Study the drawing (mm; zero at the part's minimum x, y, z) and answer. A direction names the side the tool comes from. Give positions to 0.01 mm unless a question says otherwise; leave off trailing zeros. Write each loop counter-clockwise with the first axis right and the second up, starting at its lowest first coordinate (ties: lowest second). Pieces come first, ordered by that corner, then holes. Notation, with made-up numbers: (-24, 28) - (13, 28) arc R27 ccw to (13, 58) - close; hole circle Ø1 at (-13.75, 57.25). An arc over 180 degrees is marked (long way). Write each question's results on one line, items separated by ' | '. Start each with the question number.
Q1. Find the intervals of material crossed by probe 1 along Y at (x, z) = (4.45, 1.9); probe 2 along Y at (x, z) = (2, 15); probe 3 along X at (y, z) = (25.65, 15.27), in increasing order.
Q2. Section A-A (z = 15.27) is taken. Determine the outline of the cut face in (x, y).
Q3. Section D-D (z = 4) is taken. Determine the outline of the cut face in (x, y).
Q4. For a pull along Y with two mould halves and no side action, classify the marked faces 1, 2 and 3 as pulls with the +Y half, pulls with the -Y half, needs draft (parallel to the pull), parting line crosses it, or undercut.
Q5. Flat-ended cylindrical pins translate along their axes: pin 1 Ø3 at (x, z) = (14, 15.27) entering from +Y; pin 2 Ø4 at (x, z) = (10.5, 14) entering from -Y; pin 3 Ø4 at (x, z) = (10, 5) entering from +Y. Find the tip coordinate at first contact, or state that the pin passes through.
Q6. For the marked faces 4, 5 and 6, determine the directions among +Z, -Z, +X, -X, +Y, -Y from which every point of the face is accessible in a straight line to the end or side of a thin tool.
Q7. Section B-B (y = 36.55) is taken. Determine the outline of the cut face in (x, z).
Q8. Section C-C (x = 4.45) is taken. Determine the outline of the cut face in (y, z).
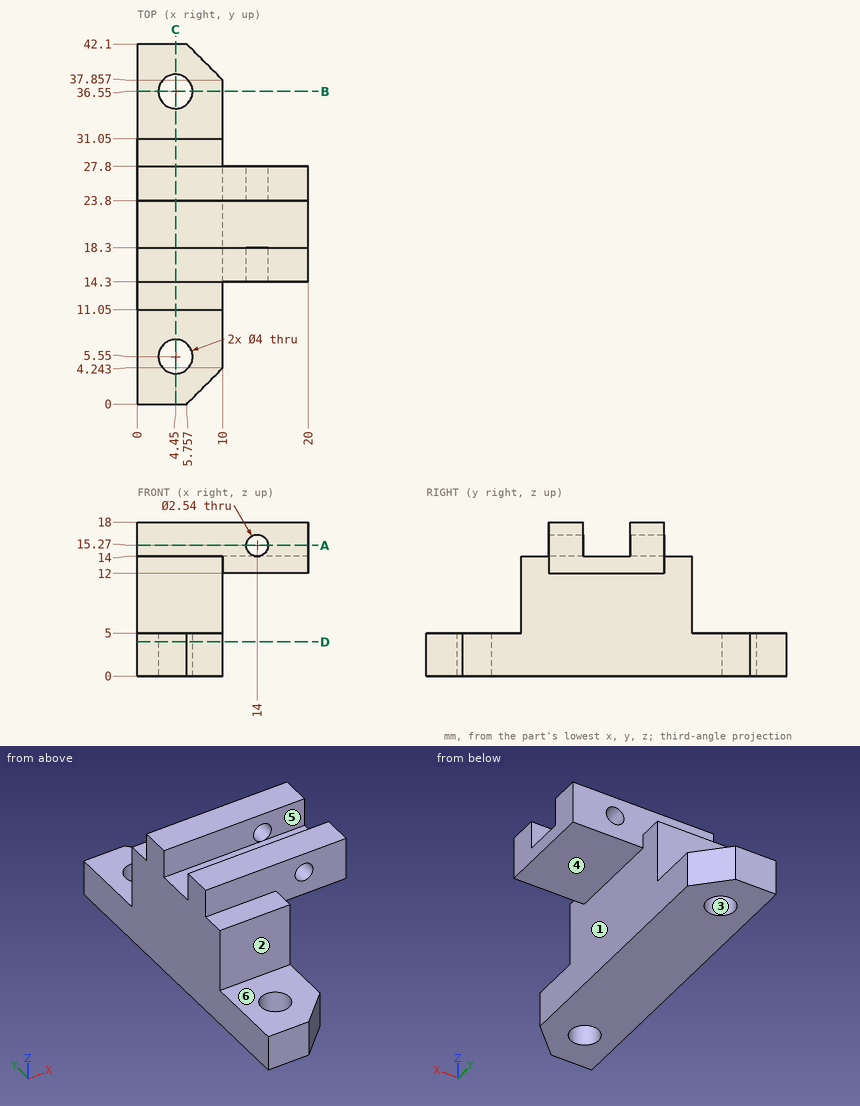
Answers below:
1) probe 1: y = 0 to 3.55, 7.55 to 34.55, 38.55 to 42.1 | probe 2: y = 14.3 to 18.3, 23.8 to 27.8 | probe 3: x = 0 to 12.73, 15.27 to 20
2) outline: (0, 14.3) - (12.73, 14.3) - (12.73, 18.3) - (0, 18.3) - close; (0, 23.8) - (12.73, 23.8) - (12.73, 27.8) - (0, 27.8) - close; (15.27, 14.3) - (20, 14.3) - (20, 18.3) - (15.27, 18.3) - close; (15.27, 23.8) - (20, 23.8) - (20, 27.8) - (15.27, 27.8) - close
3) outline: (0, 0) - (5.76, 0) - (10, 4.24) - (10, 37.86) - (5.76, 42.1) - (0, 42.1) - close; hole circle Ø4 at (4.45, 5.55); hole circle Ø4 at (4.45, 36.55)
4) face 1: needs draft | face 2: pulls with the -Y half | face 3: undercut
5) pin 1: stops at y = 27.8 | pin 2: stops at y = 11.05 | pin 3: stops at y = 39.86
6) face 4: -Z, +X, +Y, -Y | face 5: +Z, +X, -X | face 6: +Z, +X, -X, -Y
7) outline: (0, 0) - (2.45, 0) - (2.45, 5) - (0, 5) - close; (6.45, 0) - (10, 0) - (10, 5) - (6.45, 5) - close
8) outline: (0, 0) - (3.55, 0) - (3.55, 5) - (0, 5) - close; (7.55, 0) - (34.55, 0) - (34.55, 5) - (31.05, 5) - (31.05, 14) - (27.8, 14) - (27.8, 18) - (23.8, 18) - (23.8, 14) - (18.3, 14) - (18.3, 18) - (14.3, 18) - (14.3, 14) - (11.05, 14) - (11.05, 5) - (7.55, 5) - close; (38.55, 0) - (42.1, 0) - (42.1, 5) - (38.55, 5) - close
